Could you check a few things on this model? Use its own coordinates, in mm. A direction names the side the tool comes from. Give positions to 0.01 mm unless a question says otherwise; leave off trailing zeros. Loops run counter-clockwise (first coordinate to the right, second up) from the corner with the lowest first, then second, coordinate; pieces in that order, holes last.
1. Thinking about a two-plate mould opening in X: for faces 3 (the flat face through (12.7, -10, -4)), 4 (the flat face through (0, 4, 0)), 5 (the cylindrical face through (0.33, 2.52, 1.57)), 6 (the cylindrical face through (-0.551, -11.09, -7.045)), which applies, +X half, -X half, draft (parallel to the pull), parting line (faces both ways), or undercut?
2. I need wall thicknesses on line 1 along Y through (x, z) = (0, 0.85); line 2 along Z through (x, y) = (-10.5, 3.25) (3 decimals); line 3 along Y through (x, z) = (-2.75, -4) (3 decimals). Which ranges of each line are inside material? Lowest first, please.
3. Imagine slicing it at D-D (y = -10). List the corners of the cut face in (x, z) for me (3 decimals).
4. For P1, Ø4, axis at x = -0.5, z = -5, coming from the +Y side (3 decimals); P2, Ø5, axis at x = 0.5, y = 6, coming from the -Z side; P3, Ø5, axis at y = 0, z = -4, coming from the -X side, each with a flat end and sliding along its axis, tell me the tip position at first contact or that it passes through.
5. Imagine slicing it at C-C (x = 3.5). List the corners of the cut face in (y, z) for me (3 decimals).
6. Imagine slicing it at A-A (x = 0). List the corners of the cut face in (y, z) for me (3 decimals).
7. For faces 1 (the flat face through (0, -11, -22.225)), 2 (the flat face through (0, -9.525, -13)), which set-ups out of +Z, -Z, +X, -X, +Y, -Y let a thin tool reach every point of the face, with its end or its side?
8. Imagine slicing it at B-B (y = 0). List the corners of the cut face in (x, z) for me (3 decimals), plus the area to 3 significant figures.
```python
from build123d import *

# Parameters (mm, degrees)
SKETCH4_W           = 25.4
SKETCH4_H           = 25.4
BOSS_EXTRUDE3_DEPTH = 3.175
SKETCH5_W           = 25.4
SKETCH5_H           = 3.175
BOSS_EXTRUDE4_DEPTH = 22.225
SKETCH6_R           = 2.54
CUT_EXTRUDE1_DEPTH  = 4.175
SKETCH7_R           = 2.54
CUT_EXTRUDE2_DEPTH  = 4.175


with BuildPart() as part:
    # Sketch4 → Boss-Extrude3 (new body)
    with BuildSketch(Plane.XY):
        Rectangle(SKETCH4_W, SKETCH4_H)
    extrude(amount=BOSS_EXTRUDE3_DEPTH)

    # Sketch5 → Boss-Extrude4 (add)
    with BuildSketch(Plane(origin=(0, 0, 0), x_dir=(-1, 0, 0), z_dir=(0, 0, -1))):
        with Locations((0, -11.1125)):
            Rectangle(SKETCH5_W, SKETCH5_H)
    extrude(amount=BOSS_EXTRUDE4_DEPTH)

    # Sketch6 → Cut-Extrude1 (cut, through all)
    with BuildSketch(Plane(origin=(0, -9.525, 0), x_dir=(1, 0, 0), z_dir=(0, 1, 0))):
        with Locations((0, 9.525)):
            Circle(SKETCH6_R)
    extrude(amount=-CUT_EXTRUDE1_DEPTH, mode=Mode.SUBTRACT)

    # Sketch7 → Cut-Extrude2 (cut, through all)
    with BuildSketch(Plane(origin=(0, 0, 0), x_dir=(-1, 0, 0), z_dir=(0, 0, -1))):
        Circle(SKETCH7_R)
    extrude(amount=-CUT_EXTRUDE2_DEPTH, mode=Mode.SUBTRACT)


solid = part.part
```
Derived:
1. face 3: +X half
1. face 4: draft
1. face 5: undercut
1. face 6: undercut
2. line 1: y = -12.7 to -2.54, 2.54 to 12.7
2. line 2: z = 0 to 3.175
2. line 3: y = -12.7 to -9.525
3. outline: (-12.7, -22.225) - (12.7, -22.225) - (12.7, 3.175) - (-12.7, 3.175) - close; hole circle Ø5.08 at (0, -9.525)
4. P1: stops at y = -9.525
4. P2: stops at z = 0
4. P3: passes through
5. outline: (-12.7, -22.225) - (-9.525, -22.225) - (-9.525, 0) - (12.7, 0) - (12.7, 3.175) - (-12.7, 3.175) - close
6. outline: (-12.7, -22.225) - (-9.525, -22.225) - (-9.525, -12.065) - (-12.7, -12.065) - close; (-12.7, -6.985) - (-9.525, -6.985) - (-9.525, 0) - (-2.54, 0) - (-2.54, 3.175) - (-12.7, 3.175) - close; (2.54, 0) - (12.7, 0) - (12.7, 3.175) - (2.54, 3.175) - close
7. face 1: -Z, +X, -X, +Y, -Y
7. face 2: -Z, +X, -X, +Y
8. outline: (-12.7, 0) - (-2.54, 0) - (-2.54, 3.175) - (-12.7, 3.175) - close; (2.54, 0) - (12.7, 0) - (12.7, 3.175) - (2.54, 3.175) - close
8. area: 64.5 mm2
